```python
from build123d import *

# Parameters (mm, degrees)
SKETCH1_W               = 15.2
SKETCH1_H               = 15.2
BOSS_EXTRUDE1_DEPTH     = 14
SKETCH2_R               = 3.925
BOSS_EXTRUDE3_DEPTH     = 19.6
SKETCH3_W               = 32
SKETCH3_H               = 57
BOSS_EXTRUDE5_DEPTH     = 5
BOSS_EXTRUDE7_DEPTH     = 57
BOSS_EXTRUDE6_DEPTH     = 3
CUT_EXTRUDE1_DEPTH      = 73.155179994
CUT_EXTRUDE1_DEPTH_BACK = 73.155179994
SKETCH11_R              = 2.5


with BuildPart() as part:
    # Sketch1 → Boss-Extrude1 (new, symmetric)
    with BuildSketch(Plane(origin=(0, 0, 0), x_dir=(1, 0, 0), z_dir=(0, 1, 0))):
        Rectangle(SKETCH1_W, SKETCH1_H)
    extrude(amount=BOSS_EXTRUDE1_DEPTH, both=True)

    # Sketch2 → Boss-Extrude3 (add)
    with BuildSketch(Plane.XY.offset(-7.6)):
        with Locations((0, -6.45)):
            Circle(SKETCH2_R)
        with Locations((0, 9.55)):
            Circle(SKETCH2_R)
    extrude(amount=-BOSS_EXTRUDE3_DEPTH)

    # Sketch3 → Boss-Extrude5 (add)
    with BuildSketch(Plane(origin=(0, 14, 0), x_dir=(1, 0, 0), z_dir=(0, 1, 0))):
        with Locations((0, -20.9)):
            Rectangle(SKETCH3_W, SKETCH3_H)
    extrude(amount=-BOSS_EXTRUDE5_DEPTH)

    # Sketch9 → Boss-Extrude7 (add)
    with BuildSketch(Plane(origin=(0, 0, -7.6), x_dir=(-1, 0, 0), z_dir=(0, 0, -1))):
        Polygon((-16, 46.1), (-16, 14), (-12, 14), (-12, 46.1), (12, 46.1), (12, 14), (16, 14), (16, 50.1), (-16, 50.1), align=None)
    extrude(amount=-BOSS_EXTRUDE7_DEPTH)

    # Sketch5 → Boss-Extrude6 (add, symmetric)
    with BuildSketch(Plane(origin=(0, 0, 0), x_dir=(0, 0, -1), z_dir=(1, 0, 0))):
        Polygon((-7.6, -6), (-7.6, 9), (-27.6, 9), align=None)
    extrude(amount=BOSS_EXTRUDE6_DEPTH, both=True)

    # Sketch11 → Cut-Extrude1 (cut, two sides: drawn at the far end of the back side and taken through both)
    with BuildSketch(Plane(origin=(0, 0, 0), x_dir=(0, 0, -1), z_dir=(1, 0, 0)).offset(-CUT_EXTRUDE1_DEPTH_BACK)):
        with Locations((-20.1, 41.9)):
            Circle(SKETCH11_R)
        with Locations((-4.5, 41.9)):
            Circle(SKETCH11_R)
    extrude(amount=CUT_EXTRUDE1_DEPTH + CUT_EXTRUDE1_DEPTH_BACK, mode=Mode.SUBTRACT)


solid = part.part
```
Design review of the part built by this model. Coordinates are the model's own, in mm. A direction names the side the tool comes from. Coordinates: 2 decimals unless noted, no trailing zeros. Loops run counter-clockwise (first coordinate to the right, second up) from the corner with the lowest first, then second, coordinate; pieces in that order, holes last.
Q1. Tool access review of faces 1 (the face through (0, 46.1, 21)), 2 (the face through (-3, 5, 13)), 3 (the face through (4, 11, -7.6)), 4 (the face through (-7.6, -2, 0)): name each direction out of +Z, -Z, +X, -X, +Y, -Y from which nothing blocks a thin tool from reaching the whole face with its end or side.
Reported:
face 1: +Z, -Z
face 2: +Z, -X, -Y
face 3: -Z
face 4: +Z, -Z, -X, -Y
Q2. The part is to be moulded in two halves that separate along X. For faces 5 (the face through (0, 14, 21)), 6 (the face through (0, 10, -27.2)), 7 (the face through (16, 30, 21)), say which applies: +X half, -X half, draft (parallel to the pull), parting line (faces both ways), or undercut.
Reported:
face 5: undercut
face 6: draft
face 7: +X half
Q3. We need section B-B on x = 0. State the section outline as (y, z) points (3 decimals), and give its area (3 significant figures).
Reported:
outline: (-14, -7.6) - (-10.375, -7.6) - (-10.375, -27.2) - (-2.525, -27.2) - (-2.525, -7.6) - (5.625, -7.6) - (5.625, -27.2) - (13.475, -27.2) - (13.475, -7.6) - (14, -7.6) - (14, 49.4) - (9, 49.4) - (9, 27.6) - (-6, 7.6) - (-14, 7.6) - close; (46.1, -7.6) - (50.1, -7.6) - (50.1, 49.4) - (46.1, 49.4) - close
area: 1,320 mm2
Q4. We need section A-A on y = 41.9. State the section outline as (x, z) points, and give its area (3 significant figures).
Reported:
outline: (-16, -7.6) - (-12, -7.6) - (-12, 2) - (-16, 2) - close; (-16, 7) - (-12, 7) - (-12, 17.6) - (-16, 17.6) - close; (-16, 22.6) - (-12, 22.6) - (-12, 49.4) - (-16, 49.4) - close; (12, -7.6) - (16, -7.6) - (16, 2) - (12, 2) - close; (12, 7) - (16, 7) - (16, 17.6) - (12, 17.6) - close; (12, 22.6) - (16, 22.6) - (16, 49.4) - (12, 49.4) - close
area: 376 mm2
Q5. To check wall thickness, follow line 1 (Z direction, x = -13, y = 41.9); line 2 (Y direction, x = 6, z = 3); line 3 (Y direction, x = 4, z = 18). State the ranges of each line that lie inside material, in increasing order.
Reported:
line 1: z = -7.6 to 2, 7 to 17.6, 22.6 to 49.4
line 2: y = -14 to 14, 46.1 to 50.1
line 3: y = 9 to 14, 46.1 to 50.1
Q6. For pin 1 (4.5 mm diameter, centred on x = -1, y = -5.5, fed in from +Z); pin 2 (4.5 mm diameter, centred on y = 41.9, z = 20.1, fed in from +X); pin 3 (5 mm diameter, centred on x = 12.5, z = 17, fed in from -Y); pin 4 (16.5 mm diameter, centred on y = -4.5, z = -2, fed in from +X), all flat-tipped, find the tip position at first contact; note any pin that passes through.
Reported:
pin 1: stops at z = 11.27
pin 2: passes through
pin 3: stops at y = 9
pin 4: stops at x = 7.6
Q7. We need section C-C on y = 34.5. State the section outline as (x, z) points, and give its area (3 significant figures).
Reported:
outline: (-16, -7.6) - (-12, -7.6) - (-12, 49.4) - (-16, 49.4) - close; (12, -7.6) - (16, -7.6) - (16, 49.4) - (12, 49.4) - close
area: 456 mm2
Q8. We need section D-D on z = 4.5. State the section outline as (x, y) points, and give its area (3 significant figures).
Reported:
outline: (-16, 9) - (-7.6, 9) - (-7.6, -14) - (7.6, -14) - (7.6, 9) - (16, 9) - (16, 39.4) - (12, 39.4) - (12, 14) - (-12, 14) - (-12, 39.4) - (-16, 39.4) - close; (-16, 44.4) - (-12, 44.4) - (-12, 46.1) - (12, 46.1) - (12, 44.4) - (16, 44.4) - (16, 50.1) - (-16, 50.1) - close
area: 854 mm2
